Check sheet for the modelled part. Datum: model origin and axes. Units: mm. Face numbers are marked on the shaded views. A direction names the side the tool comes from. Coordinates: 2 decimals unless noted, no trailing zeros. Order: outer loops, then holes, each group sorted by start corner. A loop starts at its lowest first (then second) coordinate and runs counter-clockwise, first axis right, second up.
1. Cross-section at B-B (z = -39.5). Enter the section's corners in (x, y), then the cut area to 3 significant figures.
2. Thickness scan on line 1 (X direction, y = 20, z = -29); line 2 (Z direction, x = 29.5, y = 4.25); line 3 (Y direction, x = 16.5, z = -6). Record the ranges inside material, lowest first.
3. Cross-section at A-A (x = 35.65). Enter the section's corners in (y, z).
4. Cross-section at C-C (x = 3.5). Enter the section's corners in (y, z), then the cut area to 3 significant figures.
5. Set-up check for the marked faces 1 and 2: record each of +Z, -Z, +X, -X, +Y, -Y from which the full face is reachable in a straight line by a thin tool's end or side.
6. Gauge pin test, flat ends, axial feed: pin 1 Ø12 at (y, z) = (14, -40.5) entering from +X; pin 2 Ø3.5 at (y, z) = (13, -38) entering from -X; pin 3 Ø0.7 at (y, z) = (6, 0) entering from -X. Record the tip position at first contact, or that the pin passes through.
7. Draft check along Z on the marked faces 3, 4 and 5. Enter one of: released by +Z, released by -Z, zero draft, split by the parting line, or undercut.
```python
from build123d import *

# Parameters (mm, degrees)
BOSS_EXTRUDE1_DEPTH  = 5
SKETCH3_R            = 1.75
SKETCH3_W            = 10.8
SKETCH3_H            = 10.8
CUT_EXTRUDE1_DEPTH   = 52.721310243
FILLET1_R            = 5.4
FILLET2_R            = 5.4
SKETCH4_W            = 35
SKETCH4_H            = 20
SKETCH4_W_2          = 23
SKETCH4_H_2          = 13
BOSS_EXTRUDE2_DEPTH  = 4.25
SKETCH5_W            = 10.6
SKETCH5_H            = 20
CUT_EXTRUDE2_DEPTH   = 52.721310243
FILLET4_R            = 4
SKETCH6_W            = 8
SKETCH6_H            = 28
BOSS_EXTRUDE3_DEPTH  = 32
SKETCH7_R            = 1.3
SKETCH7_R_2          = 2.5
CUT_EXTRUDE3_DEPTH   = 32
FILLET5_R            = 8
BOSS_EXTRUDE4_DEPTH  = 8
SKETCH9_W            = 14
SKETCH9_H            = 7
CUT_EXTRUDE4_DEPTH   = 7
FILLET6_R            = 3.5
FILLET7_R            = 3.5
CUT_EXTRUDE5_DEPTH   = 8
FILLET8_R            = 4
BOSS_EXTRUDE6_START  = -9.25
BOSS_EXTRUDE6_DEPTH  = 9.25
SKETCH13_W           = 5.3
SKETCH13_H           = 13
SKETCH13_R           = 1.15
BOSS_EXTRUDE9_DEPTH  = 4.25
SKETCH14_R           = 1.35
CUT_EXTRUDE6_DEPTH   = 4.25
SKETCH15_W           = 7
SKETCH15_H           = 20
BOSS_EXTRUDE10_DEPTH = 9.25
FILLET11_R           = 5
FILLET12_R           = 2
SKETCH16_W           = 5.3
SKETCH16_H           = 13
CUT_EXTRUDE7_DEPTH   = 4.25


# Some blends are built 0.0001 mm under size
with BuildPart() as part:
    # Sketch2 → Boss-Extrude1 (new body)
    with BuildSketch(Plane(origin=(0, 0, 0), x_dir=(1, 0, 0), z_dir=(0, 1, 0))):
        Polygon((-15.080737936, 5.050942453), (-4.998489886, 19.998489886), (11.001510114, 19.998489886), (21, 10), (45, 10), (45, -10), (20.844876991, -10), (10.843650133, -25.001878594), (-5.156349867, -25.001878594), (-15.080737936, -9.949057547), align=None)
    extrude(amount=BOSS_EXTRUDE1_DEPTH)

    # Sketch3 → Cut-Extrude1 (cut, through all)
    with BuildSketch(Plane(origin=(0, 5, 0), x_dir=(1, 0, 0), z_dir=(0, 1, 0))):
        with Locations(Location((-10.080737936, 0, 0), (0, 0, 270))):
            Circle(SKETCH3_R)
        with Locations(Location((-2.117930473, -20.001878594, 0), (0, 0, 270))):
            Circle(SKETCH3_R)
        with Locations(Location((7.882069527, -20.001878594, 0), (0, 0, 270))):
            Circle(SKETCH3_R)
        with Locations((16.9, 0)):
            Rectangle(SKETCH3_W, SKETCH3_H)
    extrude(amount=-CUT_EXTRUDE1_DEPTH, mode=Mode.SUBTRACT)

    # Fillet1
    fillet1_edges = [part.edges().sort_by_distance(p)[0] for p in [
        (11.5, 2.5, 5.4),
        (11.5, 2.5, -5.4),
    ]]
    fillet(fillet1_edges, radius=FILLET1_R - 0.0001)  # a hair under: the kernel refuses the full size

    # Fillet2
    # the kernel refuses this fillet: 5.4 mm, written as the material it adds along each edge
    with BuildSketch(Plane(origin=(22.3, 5, -5.4), x_dir=(0, 0, 1), z_dir=(0, -1, 0)), Plane(origin=(22.3, 5, 5.4), x_dir=(-1, 0, 0), z_dir=(0, -1, 0))) as fillet2_piece_1:
        with BuildLine():
            CenterArc((FILLET2_R, FILLET2_R), FILLET2_R, 180, 90)
            Line((0, FILLET2_R), (0, 0))
            Line((0, 0), (FILLET2_R, 0))
        make_face()
    extrude(amount=5)
    # the kernel refuses this fillet: 5.4 mm, written as the material it takes off along each edge

    # Sketch4 → Boss-Extrude2 (add)
    with BuildSketch(Plane(origin=(0, 5, 0), x_dir=(1, 0, 0), z_dir=(0, 1, 0))):
        with Locations((16.9, 0)):
            Rectangle(SKETCH4_W, SKETCH4_H)
        with Locations((16.9, 0)):
            Rectangle(SKETCH4_W_2, SKETCH4_H_2, mode=Mode.SUBTRACT)
    extrude(amount=BOSS_EXTRUDE2_DEPTH)

    # Sketch5 → Cut-Extrude2 (cut, through all)
    with BuildSketch(Plane(origin=(0, 5, 0), x_dir=(1, 0, 0), z_dir=(0, 1, 0))):
        with Locations((39.7, 0)):
            Rectangle(SKETCH5_W, SKETCH5_H)
    extrude(amount=-CUT_EXTRUDE2_DEPTH, mode=Mode.SUBTRACT)

    # Fillet4
    fillet4_edges = [part.edges().sort_by_distance(p)[0] for p in [
        (34.4, 4.625, 10),
        (34.4, 4.625, -10),
    ]]
    fillet(fillet4_edges, radius=FILLET4_R)

    # Sketch6 → Boss-Extrude3 (add)
    with BuildSketch(Plane(origin=(0, 0, -19.998489886), x_dir=(-1, 0, 0), z_dir=(0, 0, -1))):
        with Locations((4.998489886, 14)):
            Rectangle(SKETCH6_W, SKETCH6_H)
    extrude(amount=BOSS_EXTRUDE3_DEPTH)

    # Sketch7 → Cut-Extrude3 (cut)
    with BuildSketch(Plane(origin=(-0.998489886, 0, 0), x_dir=(0, 0, -1), z_dir=(1, 0, 0))):
        with Locations(Location((33.498489886, 14, 0), (0, 0, 90))):
            Circle(SKETCH7_R)
        with Locations(Location((37.998489886, 14, 0), (0, 0, 90))):
            Circle(SKETCH7_R_2)
        with Locations(Location((42.498489886, 14, 0), (0, 0, 90))):
            Circle(SKETCH7_R)
    extrude(amount=-CUT_EXTRUDE3_DEPTH, mode=Mode.SUBTRACT)

    # Fillet5
    fillet5_edges = [part.edges().sort_by_distance(p)[0] for p in [
        (-4.998489886, 0, -51.998489886),
        (-4.998489886, 28, -51.998489886),
    ]]
    fillet(fillet5_edges, radius=FILLET5_R)

    # Sketch8 → Boss-Extrude4 (add)
    with BuildSketch(Plane(origin=(-0.998489886, 0, 0), x_dir=(0, 0, -1), z_dir=(1, 0, 0))):
        Polygon((10, 5), (10, 9.25), (19.998489886, 28), (19.998489886, 5), (19.998489886, 0), (10, 0), align=None)
    extrude(amount=-BOSS_EXTRUDE4_DEPTH)

    # Sketch9 → Cut-Extrude4 (cut)
    with BuildSketch(Plane.ZY.offset(8.998489886)):
        with Locations((-37.998489886, 14)):
            Rectangle(SKETCH9_W, SKETCH9_H)
    extrude(amount=-CUT_EXTRUDE4_DEPTH, mode=Mode.SUBTRACT)

    # Fillet6
    fillet6_edges = [part.edges().sort_by_distance(p)[0] for p in [
        (-5.498489886, 10.5, -44.998489886),
        (-5.498489886, 17.5, -44.998489886),
    ]]
    fillet(fillet6_edges, radius=FILLET6_R - 0.0001)  # a hair under: the kernel refuses the full size

    # Fillet7
    fillet7_edges = [part.edges().sort_by_distance(p)[0] for p in [
        (-5.498489886, 17.5, -30.998489886),
        (-5.498489886, 10.5, -30.998489886),
    ]]
    fillet(fillet7_edges, radius=FILLET7_R - 0.0001)  # a hair under: the kernel refuses the full size

    # Sketch10 → Cut-Extrude5 (cut)
    with BuildSketch(Plane.ZY.offset(8.998489886)):
        Polygon((-19.998489886, 28), (-10, 9.25), (-29.998489886, 28), align=None)
    extrude(amount=-CUT_EXTRUDE5_DEPTH, mode=Mode.SUBTRACT)

    # Fillet8
    fillet8_edges = [part.edges().sort_by_distance(p)[0] for p in [
        (-15.080737936, 2.5, -5.050942453),
        (11.001510114, 2.5, -19.998489886),
        (21, 2.5, -10),
        (20.844876991, 2.5, 10),
        (10.843650133, 2.5, 25.001878594),
        (-5.156349867, 2.5, 25.001878594),
        (-15.080737936, 2.5, 9.949057547),
        (-8.998489886, 2.5, -14.068246012),
        (-4.998489886, 28, -29.998489886),
    ]]
    fillet(fillet8_edges, radius=FILLET8_R)

    # Sketch12 → Boss-Extrude6 (add)
    with BuildSketch(Plane(origin=(0, 9.25, 0), x_dir=(1, 0, 0), z_dir=(0, 1, 0)).offset(BOSS_EXTRUDE6_START)):
        with BuildLine():
            Line((34.4, -6), (34.4, 6))
            ThreePointArc((34.4, 6), (33.228427125, 8.828427125), (30.4, 10))
            Line((30.4, 10), (38.3, 10))
            Line((38.3, 10), (38.3, -10))
            Line((38.3, -10), (30.4, -10))
            ThreePointArc((30.4, -10), (33.228427125, -8.828427125), (34.4, -6))
        make_face()
    extrude(amount=BOSS_EXTRUDE6_DEPTH)

    # Sketch13 → Boss-Extrude9 (add)
    with BuildSketch(Plane(origin=(0, 9.25, 0), x_dir=(1, 0, 0), z_dir=(0, 1, 0))):
        with Locations((8.05, 0)):
            Rectangle(SKETCH13_W, SKETCH13_H)
        with Locations(Location((8.05, 0, 0), (0, 0, 270))):
            Circle(SKETCH13_R, mode=Mode.SUBTRACT)
    extrude(amount=-BOSS_EXTRUDE9_DEPTH)

    # Sketch14 → Cut-Extrude6 (cut)
    with BuildSketch(Plane(origin=(0, 9.25, 0), x_dir=(1, 0, 0), z_dir=(0, 1, 0))):
        with Locations(Location((35.65, 0, 0), (0, 0, 270))):
            Circle(SKETCH14_R)
    extrude(amount=-CUT_EXTRUDE6_DEPTH, mode=Mode.SUBTRACT)

    # Sketch15 → Boss-Extrude10 (add)
    with BuildSketch(Plane(origin=(0, 9.25, 0), x_dir=(1, 0, 0), z_dir=(0, 1, 0))):
        with Locations((41.8, 0)):
            Rectangle(SKETCH15_W, SKETCH15_H)
    extrude(amount=-BOSS_EXTRUDE10_DEPTH)

    # Fillet11
    fillet11_edges = [part.edges().sort_by_distance(p)[0] for p in [
        (45.3, 4.625, -10),
        (45.3, 4.625, 10),
    ]]
    fillet(fillet11_edges, radius=FILLET11_R)

    # Fillet12
    fillet12_edges = [part.edges().sort_by_distance(p)[0] for p in [
        (-0.998489886, 18.084022871, -19.422246242),
        (-0.998489886, 27.719689703, -30.109343993),
        (-0.998489886, 28, -37.789428414),
        (-0.998489886, 25.656854249, -49.655344135),
        (-0.998489886, 0, -31.998489886),
        (-0.998489886, 2.343145751, -49.655344135),
        (19.85, 9.25, 10),
        (43.835533906, 0, 8.535533906),
        (43.835533906, 9.25, 8.535533906),
        (45.3, 9.25, 0),
        (45.3, 0, 0),
        (43.835533906, 0, -8.535533906),
        (43.835533906, 9.25, -8.535533906),
        (4.173082989, 0, -19.998489886),
        (10.875389594, 0, -19.694008016),
        (16.000755057, 0, -14.999244943),
        (21.12612052, 0, -10.30448187),
        (31.478427125, 0, -10),
        (-8.998489886, 18.084022871, -19.422246242),
        (-8.998489886, 27.719689703, -30.109343993),
        (-8.998489886, 28, -37.789428414),
        (-8.998489886, 25.656854249, -49.655344135),
        (-8.998489886, 14, -51.998489886),
        (-8.998489886, 2.343145751, -49.655344135),
        (-8.998489886, 0, -29.644829312),
        (-9.173270862, 0, -14.121681919),
        (-12.039613911, 0, -9.559594232),
        (-14.905956959, 0, -4.997506546),
        (-15.080737936, 0, 2.460546613),
        (-14.912057682, 0, 9.898455808),
        (-10.381093541, 0, 17.077245761),
        (-4.898882191, 0, 24.523738894),
        (2.850236962, 0, 25.001878594),
        (10.590345847, 0, 24.528575877),
        (15.844263562, 0, 17.500939297),
        (21.098181276, 0, 10.473302717),
        (31.642807528, 0, 10),
        (-0.998489886, 14, -51.998489886),
        (-0.6, 9.25, 0),
        (19.85, 9.25, -10),
    ]]
    fillet(fillet12_edges, radius=FILLET12_R)

    # Sketch16 → Cut-Extrude7 (cut)
    with BuildSketch(Plane(origin=(0, 9.25, 0), x_dir=(1, 0, 0), z_dir=(0, 1, 0))):
        with Locations((31.05, 0)):
            Rectangle(SKETCH16_W, SKETCH16_H)
    extrude(amount=-CUT_EXTRUDE7_DEPTH, mode=Mode.SUBTRACT)


solid = part.part
```
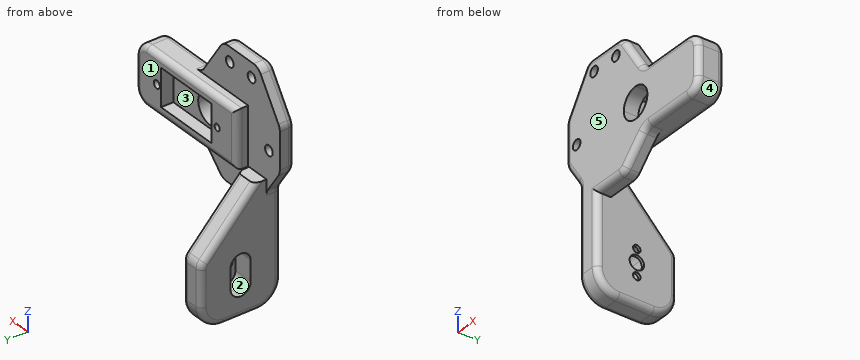
Data:
1. outline: (-9, 2) arc R2 ccw to (-7, 0) - (-3, 0) arc R2 ccw to (-1, 2) - (-1, 12) - (-2, 12) - (-2, 10.5) - (-9, 10.5) - close; (-9, 17.5) - (-2, 17.5) - (-2, 16) - (-1, 16) - (-1, 26) arc R2 ccw to (-3, 28) - (-7, 28) arc R2 ccw to (-9, 26) - close
1. area: 168 mm2
2. line 1: x = -9 to -1
2. line 2: z = -10 to 10
2. line 3: y = 0 to 5
3. outline: (0, -8) arc R2 ccw to (2, -10) - (7.25, -10) arc R2 ccw to (9.25, -8) - (9.25, -1.35) - (5, -1.35) - (5, 1.35) - (9.25, 1.35) - (9.25, 8) arc R2 ccw to (7.25, 10) - (2, 10) arc R2 ccw to (0, 8) - close
4. outline: (0, -18) arc R2 ccw to (2, -20) - (5, -20) - (5, -10) - (7.25, -10) arc R2 ccw to (9.25, -8) - (9.25, 8) arc R2 ccw to (7.25, 10) - (5, 10) - (5, 25) - (2, 25) arc R2 ccw to (0, 23) - close
4. area: 307 mm2
5. face 1: +Z, -Z, +X, -X, +Y
5. face 2: -X
6. pin 1: stops at x = -1
6. pin 2: stops at x = -2
6. pin 3: stops at x = -0.6
7. face 3: undercut
7. face 4: released by -Z
7. face 5: zero draft
